Work out the finished part from the listing and answer in its coordinate system (mm). Coordinates: 2 decimals unless noted, no trailing zeros. Write each loop counter-clockwise with the first axis right and the second up, starting at its lowest first coordinate (ties: lowest second). Pieces come first, ordered by that corner, then holes. Notation, with made-up numbers: (30, 47.25) - (43, 47.25) arc R21 cw to (43, 65.25) - close; hole circle Ø5 at (29.25, -36). An arc over 180 degrees is marked (long way). Use one line per item in the form item = value. Start each with the question number.
Item 1: Determine the mould class of faces 1 (the cylindrical face through (63.49, -7.15, 2.03)), 2 (the cylindrical face through (-63.65, 6.99, 2.03)), 3 (the cylindrical face through (-62.494, 0.264, 2.028)) for opening direction Y: released by +Y, released by -Y, zero draft, split by the parting line, or undercut.
Item 2: A cutting plane is placed at B-B (y = -4.5). Write down the section's boundary in (x, z), then the cut area to 3 significant figures.
Item 3: A cutting plane is placed at C-C (x = 52). Write down the section's boundary in (y, z).
Item 4: Consider probe 1 along Y at (x, z) = (-56.5, 1.7); probe 2 along X at (y, z) = (-0.5, 2.05); probe 3 along X at (y, z) = (8, 1.85). Determine where each line is inside the solid, lowest interval first.
Item 5: A cutting plane is placed at A-A (z = 1.85). Give the number of separate pieces and of enclosed holes in the cut face, then the cut area to 3 significant figures.
Item 6: Given pin 1 (3 mm diameter, centred on x = 4, y = 6.5, fed in from -Z); pin 2 (1 mm diameter, centred on x = 53, y = -0.5, fed in from +Z), each flat-ended and moving along its own axis, determine where each tip first touches the part or whether it passes through.
Item 7: A cutting plane is placed at D-D (y = 3.25). Write down the section's boundary in (x, z), then the cut area to 3 significant figures.
from build123d import *

# Parameters (mm, degrees)
F0_W     = 133
F0_H     = 20
F1_DEPTH = 4
F2_R     = 6
F3_DEPTH = 4.001
F4_R     = 9.99999


# Not quite as in the source:
# - a fillet or chamfer is up to 0.001 mm smaller than in the source, because OpenCascade refuses the exact size


with BuildPart() as f1:
    # F0 (on Top) → F1 (new body)
    with BuildSketch(Plane.XY):
        Rectangle(F0_W, F0_H)
    extrude(amount=F1_DEPTH)

    # F2 (on face) → F3 (cut, through all)
    with BuildSketch(Plane.XY.offset(4)):
        with Locations((-56.5, 0)):
            Circle(F2_R)
        with Locations((56.5, 0)):
            Circle(F2_R)
    extrude(amount=-F3_DEPTH, mode=Mode.SUBTRACT)

    # F4 (radius 10 in the source; OpenCascade refuses exactly that, so slightly less here)
    f4_edges = [f1.edges().sort_by_distance(p)[0] for p in [
        (-66.5, -10, 2),
        (-66.5, 10, 2),
        (66.5, -10, 2),
        (66.5, 10, 2),
    ]]
    fillet(f4_edges, radius=F4_R)


solid = f1.part
Answer:
q1.face_1 = released by -Y
q1.face_2 = released by +Y
q1.face_3 = undercut
q2.outline = (-65.43, 0) - (-60.47, 0) - (-60.47, 4) - (-65.43, 4) - close; (-52.53, 0) - (52.53, 0) - (52.53, 4) - (-52.53, 4) - close; (60.47, 0) - (65.43, 0) - (65.43, 4) - (60.47, 4) - close
q2.area = 460 mm²
q3.outline = (-10, 0) - (-3.97, 0) - (-3.97, 4) - (-10, 4) - close; (3.97, 0) - (10, 0) - (10, 4) - (3.97, 4) - close
q4.probe_1 = -10 to -6, 6 to 10
q4.probe_2 = -66.49 to -62.48, -50.52 to 50.52, 62.48 to 66.49
q4.probe_3 = -62.5 to 62.5
q5.separate_pieces = 1
q5.enclosed_holes = 2
q5.area = 2,350 mm²
q6.pin_1 = 0
q6.pin_2 = through
q7.outline = (-65.96, 0) - (-61.54, 0) - (-61.54, 4) - (-65.96, 4) - close; (-51.46, 0) - (51.46, 0) - (51.46, 4) - (-51.46, 4) - close; (61.54, 0) - (65.96, 0) - (65.96, 4) - (61.54, 4) - close
q7.area = 447 mm²
